Input: part model. Units: mm. Frame: model coordinates. A direction names the side the tool comes from. Give positions to 0.01 mm unless a question says otherwise; leave off trailing zeros. Write each loop counter-clockwise with the first axis right and the second up, starting at its lowest first coordinate (ties: lowest second). Pieces come first, ordered by that corner, then holes.
```python
from build123d import *

# Parameters (mm, degrees)
F0_R     = 9.525
F1_DEPTH = 25.4
F3_DEPTH = 12.7
F4_R     = 12.7
F5_DEPTH = 76.2
F6_R     = 3.81


with BuildPart() as f1:
    # F0 (on Front) → F1 (new body)
    with BuildSketch(Plane.XZ):
        with BuildLine():
            Line((38.1, 25.4), (0, 25.4))
            ThreePointArc((0, 25.4), (-25.4, 0), (0, -25.4))
            Line((0, -25.4), (38.1, -25.4))
            Line((38.1, -25.4), (38.1, 25.4))
        make_face()
        Circle(F0_R, mode=Mode.SUBTRACT)
    extrude(amount=F1_DEPTH)

    # F2 (on face) → F3 (join)
    with BuildSketch(Plane.YZ.offset(38.1)):
        Polygon((12.7, 25.4), (0, 25.4), (-25.4, 25.4), (-38.1, 25.4), (-38.1, -25.4), (-25.4, -25.4), (0, -25.4), (12.7, -25.4), align=None)
    extrude(amount=F3_DEPTH)

    # F4 (on face) → F5 (join)
    with BuildSketch(Plane.YZ.offset(50.8)):
        with Locations((-12.7, 0)):
            Circle(F4_R)
    extrude(amount=F5_DEPTH)

    # F6
    f6_edges = [f1.edges().sort_by_distance(p)[0] for p in [
        (127, -25.4, 0),
        (50.8, -25.4, 0),
    ]]
    fillet(f6_edges, radius=F6_R)


solid = f1.part
```
Item 1: Section A-A (z = 0). Return loops of the section in (x, y) (3 decimals).
Item 2: Section B-B (y = -12.7). Return loops of the section in (x, z) (3 decimals), and give its area (3 significant figures).
Item 3: Ray query, line 1 (X direction, y = -31.5, z = -2); line 2 (Z direction, x = 0, y = -15) (3 decimals); line 3 (Y direction, x = 30.5, z = 5). Return the intervals inside material, ascending.
Item 4: Set-up query: faces 4 (the flat face through (13, 0, 0)), 5 (the flat face through (31, -12, 25.4)), 6 (the cylindrical face through (-25.394, -12.522, 0.559)), 7 (the flat face through (38.1, -32, 0)), 8 (the flat face through (50.8, -13, 17)). Return all of +Z, -Z, +X, -X, +Y, -Y with unobstructed straight access to the full face (end or side cutting, diameter ignored); none if empty.
Item 5: Mould query, pull axis X, two halves, no side actions, for faces 1 (the flat face through (44, -38.1, 0)), 2 (the cylindrical face through (-7.559, -12.522, -5.796)), 3 (the flat face through (38.1, 6, 0)). Classes: +X half, -X half, draft (parallel to the pull), parting line (faces both ways), or undercut.
Item 6: Section C-C (x = 91). Return loops of the section in (y, z), and give its area (3 significant figures).
Item 7: Section D-D (z = 21.5). Return loops of the section in (x, y), and give its area (3 significant figures).
Item 8: Pin query (flat end, axial travel): pin 1 (6 mm diameter, centred on x = 56.5, y = -8.5, fed in from -Z); pin 2 (8 mm diameter, centred on x = 99, y = -14.5, fed in from -Z); pin 3 (1.5 mm diameter, centred on y = 4.5, z = -10.5, fed in from -X); pin 4 (15 mm diameter, centred on y = -16, z = -8.5, fed in from +X). Return the tip coordinate at first contact, or that it passes through.
Solved:
1. outline: (-25.4, -25.4) - (-9.525, -25.4) - (-9.525, 0) - (-25.4, 0) - close; (9.525, -25.4) - (38.1, -25.4) - (38.1, -38.1) - (50.8, -38.1) - (50.8, -29.21) arc R3.81 cw to (54.61, -25.4) - (123.19, -25.4) arc R3.81 ccw to (127, -21.59) - (127, -3.81) arc R3.81 ccw to (123.19, 0) - (54.61, 0) arc R3.81 cw to (50.8, 3.81) - (50.8, 12.7) - (38.1, 12.7) - (38.1, 0) - (9.525, 0) - close
2. outline: (0, -25.4) - (50.8, -25.4) - (50.8, -16.51) arc R3.81 cw to (54.61, -12.7) - (123.19, -12.7) arc R3.81 ccw to (127, -8.89) - (127, 8.89) arc R3.81 ccw to (123.19, 12.7) - (54.61, 12.7) arc R3.81 cw to (50.8, 16.51) - (50.8, 25.4) - (0, 25.4) arc R25.4 ccw to start; hole circle Ø19.05 at (0, 0)
2. area: 5,240 mm2
3. line 1: x = 38.1 to 50.8
3. line 2: z = -25.4 to -9.525, 9.525 to 25.4
3. line 3: y = -25.4 to 0
4. face 4: +Z, -Z, -X, +Y
4. face 5: +Z, +X, -X, +Y, -Y
4. face 6: -X, +Y, -Y
4. face 7: +Z, -Z, -X, -Y
4. face 8: +X
5. face 1: draft
5. face 2: undercut
5. face 3: -X half
6. outline: circle Ø25.4 at (-12.7, 0)
6. area: 507 mm2
7. outline: (-13.52, -25.4) - (38.1, -25.4) - (38.1, -38.1) - (50.8, -38.1) - (50.8, 12.7) - (38.1, 12.7) - (38.1, 0) - (-13.52, 0) - close
7. area: 1,960 mm2
8. pin 1: stops at z = -12.64
8. pin 2: stops at z = -12.7
8. pin 3: stops at x = 38.1
8. pin 4: stops at x = 127
